Design review of the part built by this model. Coordinates are the model's own, in mm. Coordinates: 2 decimals unless noted, no trailing zeros. Loops run counter-clockwise (first coordinate to the right, second up) from the corner with the lowest first, then second, coordinate; pieces in that order, holes last. Notation, with made-up numbers: (18.5, -35.5) -> (63.5, -35.5) arc R17 cw to (63.5, -28.5) -> close; hole circle Ø3 at (72.5, -24.75). An arc over 180 degrees is marked (long way). Answer as a JSON object with one key per item and string values.
Autodesk Inventor part; units mm, degrees
ref_plane "YZ Plane" through (0, 0, 0) normal (1, 0, 0) x (0, 1, 0)
ref_plane "XZ Plane" through (0, 0, 0) normal (0, 1, 0) x (-1, 0, 0)
ref_plane "XY Plane" through (0, 0, 0) normal (0, 0, 1) x (1, 0, 0)
sketch "Sketch1" plane through (0, 0, 0) normal (0, 1, 0) x (-1, 0, 0)
  line L0 (0, 0) -> (15, 0)
  line L1 (15, 0) -> (15, -99)
  line L2 (15, -99) -> (0, -99)
  line L3 (0, -99) -> (0, 0)
  circle A0 centre (4, -8) radius 1.75
  circle A1 centre (4, -91) radius 1.75
  dimension "d0" = 99
  dimension "d1" = 15
  dimension "d2" = 8
  dimension "d3" = 83
  dimension "d4" = 4
  dimension "d5" = 4
  dimension "d6" = 3.5
  dimension "d7" = 3.5
extrude "Extrusion1" add sketch "Sketch1" along normal blind 3
sketch "Sketch2" plane through (-15, 0, 0) normal (0, 0, 1) x (1, 0, 0)
  line L0 (0, 0) -> (3, 3)
  line L1 (0, 0) -> (15, 0)
  line L2 (0, 3) -> (15, 3)
  line L3 (3, 3) -> (0, 3)
  line L4 (0, 3) -> (0, 0)
  dimension "d10" = 45
extrude "Extrusion2" cut sketch "Sketch2" against normal up to surface (99 mm away)
properties part number "Cuchilla Versión 1"
1) Clearance check with a flat-ended pin moving along its axis: pin 1 Ø2 at (x, z) = (-4, -8) entering from -Y. State where the tip first meets the part, or that it passes through.
Completed:
{"pin 1": "through"}
2) Add section D-D, the plane z = -31.5. Give the boundary of the cut face in (x, y).
Completed:
{"outline": "(-15, 0) -> (0, 0) -> (0, 3) -> (-12, 3) -> close"}
3) The part is to be moulded in two halves that separate along Z. For faces 1 (the flat face through (0, 1, -50)), 2 (the flat face through (-8, 1, -99)), 3 (the cylindrical face through (-3.62, 1.48, -89.29)), 4 (the cylindrical face through (-2.71, 1.48, -9.18)), say which applies: pulls with the +Z half, pulls with the -Z half, needs draft (parallel to the pull), parting line crosses it, or undercut.
Completed:
{"face 1": "needs draft", "face 2": "pulls with the -Z half", "face 3": "undercut", "face 4": "undercut"}
4) Add section B-B, the plane z = -8. Give the boundary of the cut face in (x, y), and give its area (3 significant figures).
Completed:
{"outline": "(-15, 0) -> (-5.75, 0) -> (-5.75, 3) -> (-12, 3) -> close; (-2.25, 0) -> (0, 0) -> (0, 3) -> (-2.25, 3) -> close", "area": "30.0 mm²"}
5) Add section A-A, the plane x = -4. Give the boundary of the cut face in (y, z).
Completed:
{"outline": "(0, -99) -> (3, -99) -> (3, -92.75) -> (0, -92.75) -> close; (0, -89.25) -> (3, -89.25) -> (3, -9.75) -> (0, -9.75) -> close; (0, -6.25) -> (3, -6.25) -> (3, 0) -> (0, 0) -> close"}
6) Add section C-C, the plane y = 0.8. Give the boundary of the cut face in (x, z), and give its area (3 significant figures).
Completed:
{"outline": "(-14.2, -99) -> (0, -99) -> (0, 0) -> (-14.2, 0) -> close; hole circle Ø3.5 at (-4, -91); hole circle Ø3.5 at (-4, -8)", "area": "1,390 mm²"}
7) Wall thickness on probe 1 along Z at (x, y) = (-4, 1.7); probe 2 along Z at (x, y) = (-5, 2.05); probe 3 along X at (y, z) = (2.05, -91): over which ranges is each line inside the solid? List them lowest first.
Completed:
{"probe 1": "-99 to -92.75, -89.25 to -9.75, -6.25 to 0", "probe 2": "-99 to -92.44, -89.56 to -9.44, -6.56 to 0", "probe 3": "-12.95 to -5.75, -2.25 to 0"}
